```python
from build123d import *

# Parameters (mm, degrees)
F0_W     = 42
F0_H     = 50
F1_DEPTH = 50
F2_T     = -2.54


with BuildPart() as f1:
    # F0 (on Top) → F1 (new body)
    with BuildSketch(Plane.XY):
        Polygon((-100, 19.444444), (-50, -30.555556), (-50, 19.444444), align=None)
        with Locations((-29, -5.555556)):
            Rectangle(F0_W, F0_H)
        Polygon((-8, 19.444444), (-8, -30.555556), (42, 19.444444), align=None)
    extrude(amount=F1_DEPTH)

    # F2
    f2_openings = [f1.faces().sort_by_distance(p)[0] for p in [
        (17, -5.555556, 25),
        (-75, -5.555556, 25),
    ]]
    offset(amount=F2_T, openings=f2_openings)


solid = f1.part
```
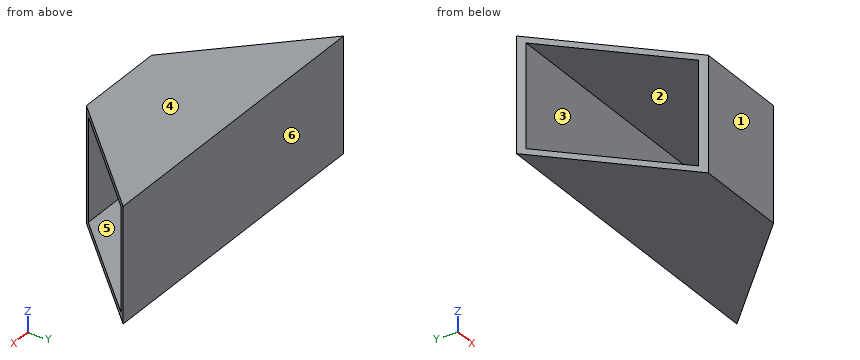
Geometry check sheet. Reference: the model listing, model coordinates, mm. Face numbers are marked on the shaded views. A direction names the side the tool comes from. Give positions to 0.01 mm unless a question says otherwise; leave off trailing zeros. Order: outer loops, then holes, each group sorted by start corner. A loop starts at its lowest first (then second) coordinate and runs counter-clockwise, first axis right, second up. Notation, with made-up numbers: (50.25, 8) - (74.25, 8) arc R17 ccw to (74.25, 30) - close; hole circle Ø4 at (64.5, 0). An arc over 180 degrees is marked (long way). Answer in a Markdown table with one row per item. Add a question column.
Q1. Mould release check, pull along Z, two halves, no side actions. Record for the marked faces 1, 2, 3 and 4: pulls with the +Z half, pulls with the -Z half, needs draft (parallel to the pull), parting line crosses it, or undercut.
Q2. Cross-section at A-A, the plane z = 23.5. Enter the section's corners in (x, y), then the cut area to 3 significant figures.
Q3. Cross-section at D-D, the plane x = -89.5. Enter the section's corners in (y, z).
Q4. Gauge pin test, flat end, axial feed: pin 1 (8 mm diameter, centred on x = 0.5, z = 25.5, fed in from -Y). Record the tip position at first contact, or that the pin passes through.
Q5. Tool access check on the marked faces 5 and 6. Record the directions out of +Z, -Z, +X, -X, +Y, -Y that give a thin tool (end or side, any length) a straight path to the whole face; none if there is none.
Q6. Cross-section at B-B, the plane y = -16.5. Enter the section's corners in (x, z).
Q7. Material ranges on probe 1 along Z at (x, y) = (-44, -24.5); probe 2 along Y at (x, z) = (-23, 17); probe 3 along Y at (x, z) = (20, 17.5), recorded low to high. Write a range as from..to.
Q8. Cross-section at C-C, the plane x = -14. Enter the section's corners in (y, z).
Check values:
| question | item | result |
|---|---|---|
| 1 | face 1 | needs draft |
| 1 | face 2 | undercut |
| 1 | face 3 | undercut |
| 1 | face 4 | pulls with the +Z half |
| 2 | outline | (-100, 19.44) - (-97.46, 16.9) - (39.46, 16.9) - (42, 19.44) - close; (-52.54, -28.02) - (-50, -30.56) - (-8, -30.56) - (-5.46, -28.02) - close |
| 2 | area | 467 mm^2 |
| 3 | outline | (8.94, 0) - (19.44, 0) - (19.44, 50) - (8.94, 50) - (8.94, 47.46) - (16.9, 47.46) - (16.9, 2.54) - (8.94, 2.54) - close |
| 4 | pin 1 | stops at y = 16.9 |
| 5 | face 5 | +X, -X |
| 5 | face 6 | +Z, -Z, +X, -X, +Y |
| 6 | outline | (-64.06, 0) - (6.06, 0) - (6.06, 2.54) - (-64.06, 2.54) - close; (-64.06, 47.46) - (6.06, 47.46) - (6.06, 50) - (-64.06, 50) - close |
| 7 | probe 1 | z = 0..2.54, 47.46..50 |
| 7 | probe 2 | y = -30.56..-28.02, 16.9..19.44 |
| 7 | probe 3 | y = 16.9..19.44 |
| 8 | outline | (-30.56, 0) - (19.44, 0) - (19.44, 50) - (-30.56, 50) - close; hole (-28.02, 2.54) - (16.9, 2.54) - (16.9, 47.46) - (-28.02, 47.46) - close |
